Read the model definition and answer for the solid it produces. Units are mm, in the model's axes. Face numbers are marked on the shaded views. Give positions to 0.01 mm unless a question says otherwise; leave off trailing zeros. Order: outer loops, then holes, each group sorted by start corner. A loop starts at its lowest first (then second) coordinate and runs counter-clockwise, first axis right, second up.
Item 1: A cutting plane is placed at A-A (x = 0). Write down the section's boundary in (y, z), plus the area to 3 significant figures.
Item 2: A cutting plane is placed at D-D (y = -28.72). Write down the section's boundary in (x, z).
Item 3: Given pin 1 Ø1.5 at (y, z) = (24.5, 2.5) entering from -X; pin 2 Ø2 at (x, z) = (-13.5, 0.5) entering from +Y, each flat-ended and moving along its own axis, determine where each tip first touches the part or whether it passes through.
Item 4: Find the intervals of material crossed by line 1 along X through (y, z) = (19, 2.4); line 2 along Y through (x, z) = (0, 1.8); line 3 along Y through (x, z) = (-15, 4.4), in increasing order.
Item 5: The mould has two halves that part along Y. Classify the marked faces 1, 2, 3 and 4: +Y half, -Y half, draft (parallel to the pull), parting line (faces both ways), or undercut.
Item 6: A cutting plane is placed at B-B (y = 19). Write down the section's boundary in (x, z), plus the area to 3 significant figures.
Item 7: A cutting plane is placed at C-C (y = 28). Write down the section's boundary in (x, z), plus the area to 3 significant figures.
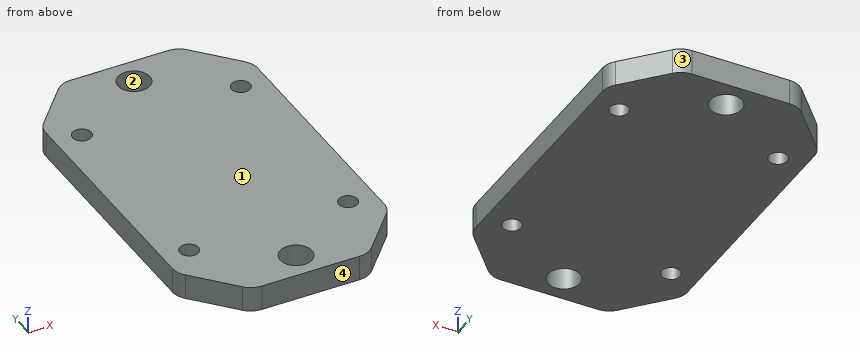
from build123d import *
from OCP.BRepFilletAPI import BRepFilletAPI_MakeChamfer

# Parameters (mm, degrees)
SKETCH1_W           = 40
SKETCH1_H           = 67.88
SKETCH1_R           = 3
SKETCH1_R_2         = 1.75
BOSS_EXTRUDE1_DEPTH = 4.7625
CHAMFER1_SIZE       = 10
CHAMFER1_SIZE2      = 9.004040443
FILLET1_R           = 4


with BuildPart() as part:
    # Sketch1 → Boss-Extrude1 (new body)
    with BuildSketch(Plane.XY):
        Rectangle(SKETCH1_W, SKETCH1_H)
        with Locations(Location((4.07e-07, 28.72, 0), (0, 0, 180))):
            Circle(SKETCH1_R, mode=Mode.SUBTRACT)
        with Locations(Location((-4.07e-07, -28.72, 0), (0, 0, 180))):
            Circle(SKETCH1_R, mode=Mode.SUBTRACT)
        with Locations(Location((-14.999999995, 19, 0), (0, 0, 180))):
            Circle(SKETCH1_R_2, mode=Mode.SUBTRACT)
        with Locations(Location((-14.999999995, -19, 0), (0, 0, 180))):
            Circle(SKETCH1_R_2, mode=Mode.SUBTRACT)
        with Locations(Location((15.000000005, 19, 0), (0, 0, 180))):
            Circle(SKETCH1_R_2, mode=Mode.SUBTRACT)
        with Locations(Location((15.000000005, -19, 0), (0, 0, 180))):
            Circle(SKETCH1_R_2, mode=Mode.SUBTRACT)
    extrude(amount=BOSS_EXTRUDE1_DEPTH)

    # Chamfer1: one chamfer whose edges measure the first distance from different faces: ONE call of the kernel's chamfer builder (chamfer() names one face for all edges)
    chamfer1_edges_1 = [part.edges().sort_by_distance(p)[0] for p in [
        (20, -33.94, 2.38125),
        (20, 33.94, 2.38125),
    ]]
    chamfer1_side_1 = [part.faces().sort_by_distance(p)[0] for p in [
        (20, 0, 2.38125),
    ]]
    chamfer1_edges_2 = [part.edges().sort_by_distance(p)[0] for p in [
        (-20, -33.94, 2.38125),
        (-20, 33.94, 2.38125),
    ]]
    chamfer1_side_2 = [part.faces().sort_by_distance(p)[0] for p in [
        (-20, 0, 2.38125),
    ]]
    chamfer1 = BRepFilletAPI_MakeChamfer(part.part.solid().wrapped)
    for e in chamfer1_edges_1:
        chamfer1.Add(CHAMFER1_SIZE, CHAMFER1_SIZE2, e.wrapped, chamfer1_side_1[0].wrapped)  # the first distance lies on this face
    for e in chamfer1_edges_2:
        chamfer1.Add(CHAMFER1_SIZE, CHAMFER1_SIZE2, e.wrapped, chamfer1_side_2[0].wrapped)  # the first distance lies on this face
    add(Compound.cast(chamfer1.Shape()), mode=Mode.REPLACE)

    # Fillet1
    fillet1_edges = [part.edges().sort_by_distance(p)[0] for p in [
        (-20, -23.94, 2.38125),
        (-20, 23.94, 2.38125),
        (10.995959557, 33.94, 2.38125),
        (-10.995959557, 33.94, 2.38125),
        (10.995959557, -33.94, 2.38125),
        (-10.995959557, -33.94, 2.38125),
        (20, -23.94, 2.38125),
        (20, 23.94, 2.38125),
    ]]
    fillet(fillet1_edges, radius=FILLET1_R)


solid = part.part
Response values:
1. outline: (-33.94, 0) - (-31.72, 0) - (-31.72, 4.76) - (-33.94, 4.76) - close; (-25.72, 0) - (25.72, 0) - (25.72, 4.76) - (-25.72, 4.76) - close; (31.72, 0) - (33.94, 0) - (33.94, 4.76) - (31.72, 4.76) - close
1. area: 266 mm2
2. outline: (-15.7, 0) - (-3, 0) - (-3, 4.76) - (-15.7, 4.76) - close; (3, 0) - (15.7, 0) - (15.7, 4.76) - (3, 4.76) - close
3. pin 1: stops at x = -19.77
3. pin 2: stops at y = 32.27
4. line 1: x = -20 to -16.75, -13.25 to 13.25, 16.75 to 20
4. line 2: y = -33.94 to -31.72, -25.72 to 25.72, 31.72 to 33.94
4. line 3: y = -29.49 to -20.75, -17.25 to 17.25, 20.75 to 29.49
5. face 1: draft
5. face 2: undercut
5. face 3: +Y half
5. face 4: -Y half
6. outline: (-20, 0) - (-16.75, 0) - (-16.75, 4.76) - (-20, 4.76) - close; (-13.25, 0) - (13.25, 0) - (13.25, 4.76) - (-13.25, 4.76) - close; (16.75, 0) - (20, 0) - (20, 4.76) - (16.75, 4.76) - close
6. area: 157 mm2
7. outline: (-16.34, 0) - (-2.91, 0) - (-2.91, 4.76) - (-16.34, 4.76) - close; (2.91, 0) - (16.34, 0) - (16.34, 4.76) - (2.91, 4.76) - close
7. area: 128 mm2
